Source: CAD feature listing. Evaluate the final solid. Frame: model axes, mm. Face numbers are marked on the shaded views. Coordinates: 2 decimals unless noted, no trailing zeros.
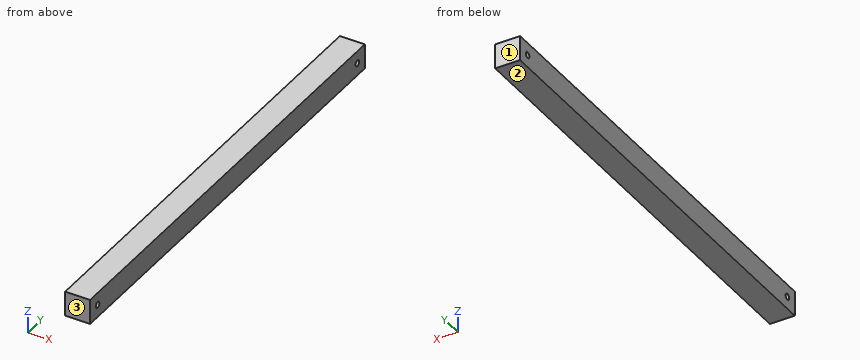
```python
from build123d import *

# Parameters (mm, degrees)
F0_W     = 63.5
F0_H     = 63.5
F1_DEPTH = 1168.4
F3_DEPTH = 25.4
F4_DEPTH = 63.5
F5_W     = 25.4
F5_H     = 63.5
F6_DEPTH = 63.5
F8_DEPTH = 76.2


with BuildPart() as f1:
    # F0 (on Front) → F1 (new body)
    with BuildSketch(Plane.XZ):
        with Locations((-65.2197142243, 64.7908774316)):
            Rectangle(F0_W, F0_H)
    extrude(amount=-F1_DEPTH)

    # F2 (on face) → F3 (join)
    with BuildSketch(Plane(origin=(-96.9697142243, 0, 0), x_dir=(0, -1, 0), z_dir=(-1, 0, 0))):
        with BuildLine():
            Line((-1168.4, 96.5408774316), (-1168.4, 33.0408774316))
            Line((-1168.4, 33.0408774316), (-1136.65, 33.0408774316))
            Line((-1136.65, 33.0408774316), (-1136.65, 57.1708774316))
            ThreePointArc((-1136.65, 57.1708774316), (-1144.27, 64.7908774316), (-1136.65, 72.4108774316))
            Line((-1136.65, 72.4108774316), (-1136.65, 96.5408774316))
            Line((-1136.65, 96.5408774316), (-1168.4, 96.5408774316))
        make_face()
        with BuildLine():
            Line((-1136.65, 57.1708774316), (-1136.65, 33.0408774316))
            Line((-1136.65, 33.0408774316), (-1104.9, 33.0408774316))
            Line((-1104.9, 33.0408774316), (-1104.9, 96.5408774316))
            Line((-1104.9, 96.5408774316), (-1136.65, 96.5408774316))
            Line((-1136.65, 96.5408774316), (-1136.65, 72.4108774316))
            ThreePointArc((-1136.65, 72.4108774316), (-1131.2618463274, 70.1790311043), (-1129.03, 64.7908774316))
            ThreePointArc((-1129.03, 64.7908774316), (-1131.2618463274, 59.402723759), (-1136.65, 57.1708774316))
        make_face()
    extrude(amount=F3_DEPTH)

    # F4 (cut): a face of the model
    f4_faces = [f1.faces().sort_by_distance(p)[0] for p in [
        (-96.9697142243, 1136.65, 64.7908774316),
    ]]
    extrude(f4_faces, amount=-F4_DEPTH, mode=Mode.SUBTRACT)

    # F5 (on face) → F6 (cut)
    with BuildSketch(Plane.XY.offset(96.5408774316)):
        with Locations((-109.6697142243, 1136.65)):
            Rectangle(F5_W, F5_H)
    extrude(amount=-F6_DEPTH, mode=Mode.SUBTRACT)

    # F7 (on face) → F8 (cut)
    with BuildSketch(Plane(origin=(-96.9697142243, 0, 0), x_dir=(0, -1, 0), z_dir=(-1, 0, 0))):
        with BuildLine():
            ThreePointArc((-24.13, 64.7908774316), (-26.3618463274, 70.1790311043), (-31.75, 72.4108774316))
            Line((-31.75, 72.4108774316), (-31.75, 57.1708774316))
            ThreePointArc((-31.75, 57.1708774316), (-26.3618463274, 59.402723759), (-24.13, 64.7908774316))
        make_face()
        with BuildLine():
            Line((-31.75, 57.1708774316), (-31.75, 72.4108774316))
            ThreePointArc((-31.75, 72.4108774316), (-39.37, 64.7908774316), (-31.75, 57.1708774316))
        make_face()
    extrude(amount=-F8_DEPTH, mode=Mode.SUBTRACT)


solid = f1.part
```
Q1. Material intervals for line 1 along Y through (x, z) = (-77.5, 62.5); line 2 along Y through (x, z) = (-83.5, 58), sorted ascending.
Solutions:
line 1: y = 0 to 24.48, 39.02 to 1129.38, 1143.92 to 1168.4
line 2: y = 0 to 28.29, 35.21 to 1133.19, 1140.11 to 1168.4
Q2. Pull-direction query (Y, two-part tool) for the marked faces 1, 2 and 3; classes: pulls with the +Y half, pulls with the -Y half, needs draft (parallel to the pull), parting line crosses it, or undercut.
Solutions:
face 1: pulls with the +Y half
face 2: needs draft
face 3: pulls with the -Y half
Q3. Pin query (flat end, axial travel): P1, Ø3, axis at x = -82.5, z = 63, coming from the -Y side. Return the tip coordinate at first contact, or that it passes through.
Solutions:
P1: stops at y = 0
